Geometry: final body of the model. Coordinates: model frame, mm. A direction names the side the tool comes from. Round coordinates to 2 decimals unless told otherwise and drop trailing zeros. Write each loop counter-clockwise with the first axis right and the second up, starting at its lowest first coordinate (ties: lowest second). Pieces come first, ordered by that corner, then holes.
Solid Edge part; units mm, degrees
sketch "Sketch1" plane through (0, 0, 0) normal (0, -1, 0) x (1, 0, 0)
  line L0 (0, -17.2662) -> (2.413, -17.2662)
  line L1 (2.413, -17.2662) -> (2.413, 1.1488)
  line L2 (2.413, 1.1488) -> (3.863, 1.1488)
  line L3 (3.863, 1.1488) -> (3.863, 5.9748)
  line L4 (3.863, 5.9748) -> (0, 5.9748)
revolve "RevolvedProtrusion1" add sketch "Sketch1" angle 360 about axis through (0, 0, 5.9748) along (0, 0, -1)
sketch "Sketch2" plane through (0, 0, 5.9748) normal (0, 0, 1) x (1, 0, 0)
  line L0 (-1.9403, 0) -> (-0.9702, 1.6804)
  line L1 (-0.9702, 1.6804) -> (0.9702, 1.6804)
  line L2 (0.9702, 1.6804) -> (1.9403, 0)
  line L3 (1.9403, 0) -> (0.9702, -1.6804)
  line L4 (0.9702, -1.6804) -> (-0.9702, -1.6804)
  line L5 (-0.9702, -1.6804) -> (-1.9403, 0)
extrude "Cutout1" cut sketch "Sketch2" against normal blind 3.2156
sketch "Sketch3" plane through (0, 0, -12.9482) normal (0, 0, -1) x (0, -1, 0)
  line L0 (4.953, 0) -> (4.953, 5.461)
  line L1 (4.953, 5.461) -> (-7.747, 5.461)
  line L2 (-7.747, 5.461) -> (-7.747, -5.461)
  line L3 (-7.747, -5.461) -> (4.953, -5.461)
  line L4 (4.953, -5.461) -> (4.953, 0)
extrude "Protrusion1" add sketch "Sketch3" along normal up to vertex (4.318 mm away)
sketch "Sketch4" plane through (0, 7.747, -15.1072) normal (0, 1, 0) x (-1, 0, 0)
  line L0 (0, -2.159) -> (3.4925, -2.159)
  line L1 (3.4925, -2.159) -> (5.461, 0.254)
  line L2 (5.461, 0.254) -> (6.5845, 0.254)
  line L3 (6.5845, -3.7102) -> (6.5845, 0.254)
  line L4 (-7.3862, -3.7102) -> (6.5845, -3.7102)
  line L5 (-7.3862, 0.254) -> (-7.3862, -3.7102)
  line L6 (-5.461, 0.254) -> (-7.3862, 0.254)
  line L7 (-5.461, 0.254) -> (-3.4925, -2.159)
  line L8 (0, -2.159) -> (-3.4925, -2.159)
extrude "ExtrudedCutout_2" cut sketch "Sketch4" against normal blind 371.1855
1) Section B-B on x = -3.25. Output: boundary loops of the cut face in (y, z).
2) Section C-C on y = -3. Output: boundary loops of the cut face in (x, z), plus the area to 3 significant figures.
3) Line query: probe 1 along Z at (x, y) = (-3.25, 1.5); probe 2 along Z at (x, y) = (1.75, 6.75); probe 3 along Z at (x, y) = (-0.75, 0). Output: solid intervals per line, ascending.
4) Section A-A on x = 0. Output: boundary loops of the cut face in (y, z), plus the area to 3 significant figures.
5) First-contact query: P1, Ø6, axis at x = -2, z = 3.5, coming from the -Y side; P2, Ø1.7, axis at x = 0, y = -0.5, coming from the +Z side; P3, Ø0.6, axis at x = 0, z = 4.5, coming from the +Y side. Flat tips, straight axial feed; report the tip coordinate or a pass-through.
6) Reachability of faces 5 (the flat face through (-2, 2, 1.149)), 6 (the flat face through (-1.46, 0.83, 4.39)), 7 (the flat face through (0, -2, 5.975)) from +Z, -Z, +X, -X, +Y, -Y: full face, straight path, thin tool, end or side. Return the list, or none.
7) Section D-D on y = 4.5. Output: boundary loops of the cut face in (x, z), plus the area to 3 significant figures.
8) Draft query along X for faces 1 (the flat face through (-5.461, 1, -14)), 2 (the flat face through (-1.45, -0.85, 4.39)), 3 (the flat face through (0, 3, -12.948)), 4 (the cylindrical face through (3.685, 1.16, 3.596)). Return one class per face: pulls with the +X half, pulls with the -X half, needs draft (parallel to the pull), parting line crosses it, or undercut.
Filled in:
1. outline: (-4.95, -17.27) - (7.75, -17.27) - (7.75, -12.95) - (-4.95, -12.95) - close; (-2.09, 1.15) - (2.09, 1.15) - (2.09, 5.97) - (-2.09, 5.97) - close
2. outline: (-5.46, -14.85) - (-3.49, -17.27) - (3.49, -17.27) - (5.46, -14.85) - (5.46, -12.95) - (-5.46, -12.95) - close; (-2.43, 1.15) - (2.43, 1.15) - (2.43, 5.97) - (-2.43, 5.97) - close
2. area: 65.9 mm2
3. probe 1: z = -17.27 to -12.95, 1.15 to 5.97
3. probe 2: z = -17.27 to -12.95
3. probe 3: z = -17.27 to 2.76
4. outline: (-4.95, -17.27) - (7.75, -17.27) - (7.75, -12.95) - (2.41, -12.95) - (2.41, 1.15) - (3.86, 1.15) - (3.86, 5.97) - (1.68, 5.97) - (1.68, 2.76) - (-1.68, 2.76) - (-1.68, 5.97) - (-3.86, 5.97) - (-3.86, 1.15) - (-2.41, 1.15) - (-2.41, -12.95) - (-4.95, -12.95) - close
4. area: 149 mm2
5. P1: stops at y = -3.86
5. P2: stops at z = 2.76
5. P3: stops at y = 3.86
6. face 5: none
6. face 6: +Z
6. face 7: +Z, +X, -X, +Y, -Y
7. outline: (-5.46, -14.85) - (-3.49, -17.27) - (3.49, -17.27) - (5.46, -14.85) - (5.46, -12.95) - (-5.46, -12.95) - close
7. area: 42.4 mm2
8. face 1: pulls with the -X half
8. face 2: undercut
8. face 3: needs draft
8. face 4: parting line crosses it
